```python
from build123d import *

# Parameters (mm, degrees)
F0_R     = 7.5
F0_R_2   = 1.5
F1_DEPTH = 5
F3_DEPTH = 25
F4_R     = 0.75
F5_DEPTH = 25


with BuildPart() as f1:
    # F0 (on Front) → F1 (new body)
    with BuildSketch(Plane.XZ):
        Circle(F0_R)
        Circle(F0_R_2, mode=Mode.SUBTRACT)
    extrude(amount=F1_DEPTH)

    # F2 (on face) → F3 (cut)
    with BuildSketch(Plane.XZ.offset(5)):
        Polygon((7.705039, 6.243331), (4.710033, 5.836573), (5.342667, -6.620519), (8.805699, -9.096223), (11.449249, 0), align=None)
        Polygon((-4.710033, -5.836573), (-5.342667, 6.620519), (-10.334909, 6.971451), (-9.518318, -9.107922), align=None)
    extrude(amount=-F3_DEPTH, mode=Mode.SUBTRACT)

    # F4 (on face) → F5 (cut)
    with BuildSketch(Plane(origin=(4.993565, 0, 0.253598), x_dir=(0, 1, 0), z_dir=(0.998713, 0, 0.05072))):
        with Locations((-2.5, 0)):
            Circle(F4_R)
    extrude(amount=-F5_DEPTH, mode=Mode.SUBTRACT)


solid = f1.part
```
Work out the finished part from the listing and answer in its coordinate system (mm). Give positions to 0.01 mm unless a question says otherwise; leave off trailing zeros. Order: outer loops, then holes, each group sorted by start corner. A loop starts at its lowest first (then second) coordinate and runs counter-clockwise, first axis right, second up.
1. Each of these flat-tipped pins is pushed along its axis until it touches: P1, Ø2, axis at y = -3.5, z = -3.5, coming from the -X side; P2, Ø1, axis at x = -2, y = -3.5, coming from the -Z side; P3, Ø2.5, axis at x = 0, z = 0, coming from the +Y side; P4, Ø1.5, axis at y = -0.5, z = -2.5, coming from the +X side. Where does it stop, or does it pass through?
Result sheet:
P1: stops at x = -4.88
P2: stops at z = -7.35
P3: passes through
P4: stops at x = 5.17
2. The mould has two halves that part along Z. Classify faces 1 (the flat face through (-4.99, -3.65, -0.33)), 2 (the flat face through (0, 0, -2)), 3 (the cylindrical face through (3.19, -3.1, -0.29)), 4 (the cylindrical face through (-3.08, -2.66, -0.89)): released by +Z, released by -Z, zero draft, split by the parting line, or undercut.
Result sheet:
face 1: released by -Z
face 2: zero draft
face 3: undercut
face 4: undercut
3. Straight lines are drawn through the part: L1, parallel to Z at x = 0, y = -3.05; L2, parallel to X at y = -1.25, z = 0; L3, parallel to Z at x = 1, y = -2.05. For each, find the intervals that lie inside material, in ascending order.
Result sheet:
L1: z = -7.5 to -1.5, 1.5 to 7.5
L2: x = -5.01 to -1.5, 1.5 to 5.01
L3: z = -7.43 to -1.12, 1.12 to 7.43
4. Section C-C, the plane y = -1.3 is taken. Determine the outline of the cut face in (x, z).
Result sheet:
outline: (-5.28, 5.33) - (-4.71, -5.84) arc R7.5 ccw to (5.28, -5.33) - (4.71, 5.84) arc R7.5 ccw to start; hole circle Ø3 at (0, 0)
5. Section A-A, the plane y = -2.9 is taken. Determine the outline of the cut face in (x, z), and give its area (3 significant figures).
Result sheet:
outline: (-5.28, 5.33) - (-5.03, 0.38) - (-1.39, 0.56) arc R1.5 cw to (1.33, 0.7) - (4.96, 0.89) - (4.71, 5.84) arc R7.5 ccw to start; (-4.96, -0.89) - (-4.71, -5.84) arc R7.5 ccw to (5.28, -5.33) - (5.03, -0.38) - (1.39, -0.56) arc R1.5 cw to (-1.33, -0.7) - close
area: 122 mm2
6. Section B-B, the plane x = 0 is taken. Determine the outline of the cut face in (y, z).
Result sheet:
outline: (-5, -7.5) - (0, -7.5) - (0, -1.5) - (-5, -1.5) - close; (-5, 1.5) - (0, 1.5) - (0, 7.5) - (-5, 7.5) - close
7. Section D-D, the plane z = 1.75 is taken. Determine the outline of the cut face in (x, y), and give its area (3 significant figures).
Result sheet:
outline: (-5.1, -5) - (4.92, -5) - (4.92, 0) - (-5.1, 0) - close
area: 50.1 mm2
